from build123d import *

# Parameters (mm, degrees)
SKETCH_1_W          = 25
SKETCH_1_H          = 50
EXTRUDE_1_DEPTH     = 5
SKETCH_2_R          = 2.25
CUT_EXTRUDE_1_DEPTH = 20
SKETCH_3_W          = 25
SKETCH_3_H          = 8
EXTRUDE_2_DEPTH     = 15
SKETCH_4_W          = 25
SKETCH_4_H          = 26
EXTRUDE_3_DEPTH     = 5
SKETCH_5_R          = 2.25
CUT_EXTRUDE_2_DEPTH = 5
SKETCH_6_W          = 25
SKETCH_6_H          = 50
CUT_EXTRUDE_3_DEPTH = 5


with BuildPart() as part:
    # 草图1 → 凸台-拉伸1 (new body)
    with BuildSketch(Plane.XY):
        with Locations((12.5, 25)):
            Rectangle(SKETCH_1_W, SKETCH_1_H)
    extrude(amount=EXTRUDE_1_DEPTH)

    # 草图2 → 切除-拉伸1 (cut)
    with BuildSketch(Plane.XY.offset(5)):
        with Locations((12.5, 7.5)):
            Circle(SKETCH_2_R)
        with Locations((12.5, 42.5)):
            Circle(SKETCH_2_R)
    extrude(amount=-CUT_EXTRUDE_1_DEPTH, mode=Mode.SUBTRACT)

    # 草图3 → 凸台-拉伸2 (add)
    with BuildSketch(Plane.XY.offset(5)):
        with Locations((12.5, 25)):
            Rectangle(SKETCH_3_W, SKETCH_3_H)
    extrude(amount=EXTRUDE_2_DEPTH)

    # 草图4 → 凸台-拉伸3 (add)
    with BuildSketch(Plane.XY.offset(20)):
        with Locations((12.5, 25)):
            Rectangle(SKETCH_4_W, SKETCH_4_H)
    extrude_3 = extrude(amount=EXTRUDE_3_DEPTH)

    # 草图5 → 切除-拉伸2 (cut)
    with BuildSketch(Plane(origin=(0, 0, 20), x_dir=(-1, 0, 0), z_dir=(0, 0, -1))):
        with Locations((-18.5, 33.5)):
            Circle(SKETCH_5_R)
        with Locations((-6.5, 33.5)):
            Circle(SKETCH_5_R)
        with Locations((-6.5, 16.5)):
            Circle(SKETCH_5_R)
        with Locations((-18.5, 16.5)):
            Circle(SKETCH_5_R)
    cut_extrude_2 = extrude(amount=-CUT_EXTRUDE_2_DEPTH, mode=Mode.SUBTRACT)

    # 草图6 → 切除-拉伸3 (cut)
    with BuildSketch(Plane(origin=(0, 0, 0), x_dir=(-1, 0, 0), z_dir=(0, 0, -1))):
        with Locations((-12.5, 25)):
            Rectangle(SKETCH_6_W, SKETCH_6_H)
    extrude(amount=-CUT_EXTRUDE_3_DEPTH, mode=Mode.SUBTRACT)

    # 镜向1: 凸台-拉伸3, 切除-拉伸2 across plane
    add(extrude_3.mirror(Plane(origin=(0, 0, 12.5), x_dir=(1, 0, 0), z_dir=(0, 0, -1))))
    add(cut_extrude_2.mirror(Plane(origin=(0, 0, 12.5), x_dir=(1, 0, 0), z_dir=(0, 0, -1))), mode=Mode.SUBTRACT)


solid = part.part
The listing builds one solid part. Answer for the finished solid, in the listing's coordinates (mm). A direction names the side the tool comes from. Round coordinates to 2 decimals unless told otherwise and drop trailing zeros. Loops run counter-clockwise (first coordinate to the right, second up) from the corner with the lowest first, then second, coordinate; pieces in that order, holes last. Notation, with made-up numbers: M 60,-15.5 L 113,-15.5 A16 cw 113,13.5 Z; hole C 52,32 d4. An arc over 180 degrees is marked long. Write each question's results on one line, items separated by ' | '. Start each with the question number.
1) Each of these flat-tipped pins is pushed along its axis until it touches: pin 1 (12 mm diameter, centred on x = 18, z = 12.5, fed in from -Y); pin 2 (4 mm diameter, centred on x = 18.5, y = 33.5, fed in from -Z); pin 3 (12 mm diameter, centred on x = 10, z = 12, fed in from +Y). Where does it stop, or does it pass through?
2) Find section C-C on y = 33.5. Write down the section's boundary in (x, z), plus the area to 3 significant figures.
3) Which of the six approach directions +Z, -Z, +X, -X, +Y, -Y give full straight-line access (tool end or side, diameter ignored) to faces 4 (the flat face through (12, 34, 20)), 5 (the cylindrical face through (6.988, 14.304, 2.535)), 6 (the flat face through (12, 17, 20))?
4) Straight lines are drawn through the part: probe 1 along Y at (x, z) = (6.5, 1.35); probe 2 along Z at (x, y) = (7.25, 30); probe 3 along Y at (x, z) = (19, 14.25). For each, find the intervals that lie inside material, in ascending order.
5) Determine the mould class of faces 1 (the flat face through (12, 25, 0)), 2 (the cylindrical face through (17.462, 14.504, 2.535)), 3 (the flat face through (12, 34, 5)) for opening direction Z: pulls with the +Z half, pulls with the -Z half, needs draft (parallel to the pull), parting line crosses it, or undercut.
6) Find section A-A on x = 18.5. Write down the section's boundary in (y, z).
7) Find section B-B on y = 36.25. Write down the section's boundary in (x, z), plus the area to 3 significant figures.
8) Find section D-D on z = 17. Write down the section's boundary in (x, y), plus the area to 3 significant figures.
Final values:
1) pin 1: y = 21 | pin 2: through | pin 3: y = 29
2) outline: M 0,0 L 4.25,0 L 4.25,5 L 0,5 Z; M 0,20 L 4.25,20 L 4.25,25 L 0,25 Z; M 8.75,0 L 16.25,0 L 16.25,5 L 8.75,5 Z; M 8.75,20 L 16.25,20 L 16.25,25 L 8.75,25 Z; M 20.75,0 L 25,0 L 25,5 L 20.75,5 Z; M 20.75,20 L 25,20 L 25,25 L 20.75,25 Z | area: 160 mm²
3) face 4: +X, -X, +Y | face 5: +Z, -Z | face 6: +X, -X, -Y
4) probe 1: 12 to 14.25, 18.75 to 31.25, 35.75 to 38 | probe 2: 0 to 5, 20 to 25 | probe 3: 21 to 29
5) face 1: pulls with the -Z half | face 2: needs draft | face 3: undercut
6) outline: M 12,0 L 14.25,0 L 14.25,5 L 12,5 Z; M 12,20 L 14.25,20 L 14.25,25 L 12,25 Z; M 18.75,0 L 31.25,0 L 31.25,5 L 29,5 L 29,20 L 31.25,20 L 31.25,25 L 18.75,25 L 18.75,20 L 21,20 L 21,5 L 18.75,5 Z; M 35.75,0 L 38,0 L 38,5 L 35.75,5 Z; M 35.75,20 L 38,20 L 38,25 L 35.75,25 Z
7) outline: M 0,0 L 25,0 L 25,5 L 0,5 Z; M 0,20 L 25,20 L 25,25 L 0,25 Z | area: 250 mm²
8) outline: M 0,21 L 25,21 L 25,29 L 0,29 Z | area: 200 mm²
